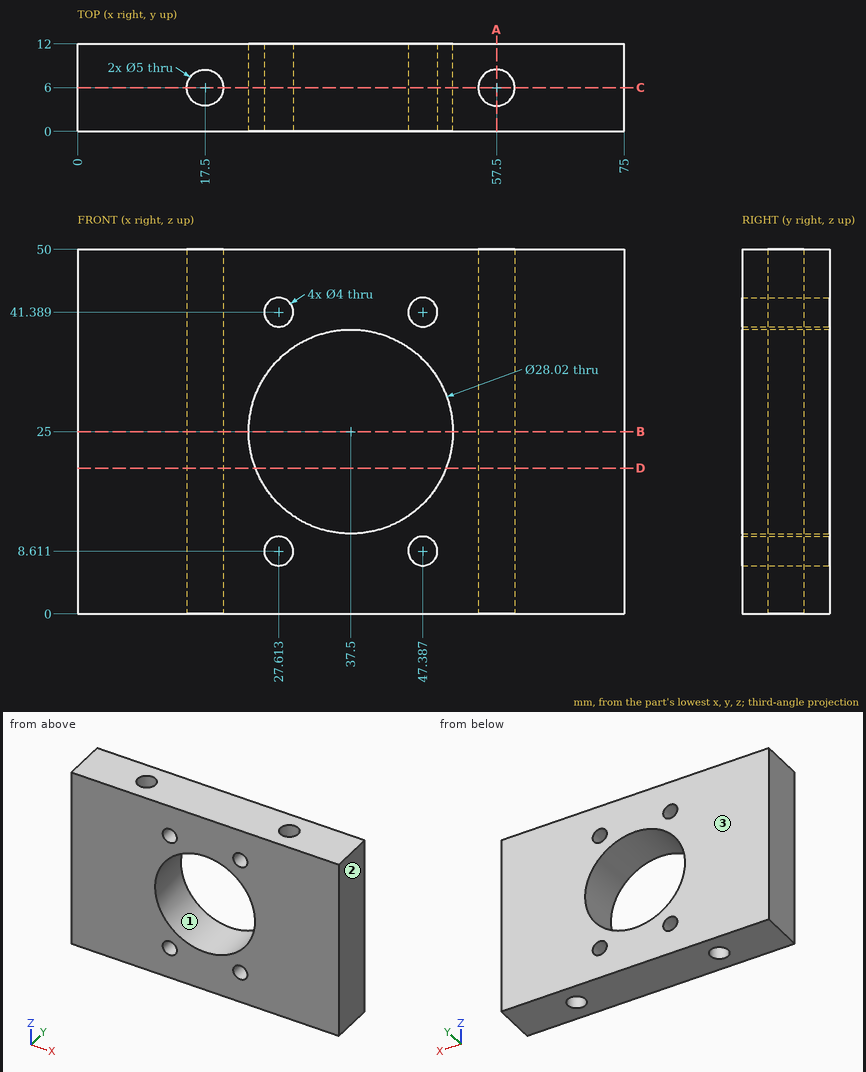
Geometry check sheet. Reference: drawing and pictorial views, mm from the part's lowest x, y, z. Round coordinates to 2 decimals unless told otherwise and drop trailing zeros. Loops run counter-clockwise (first coordinate to the right, second up) from the corner with the lowest first, then second, coordinate; pieces in that order, holes last. Notation, with made-up numbers: (34, 48.5) - (92, 48.5) arc R27 cw to (92, 82.5) - close; hole circle Ø9 at (-6.5, -33). An arc over 180 degrees is marked (long way). Answer in a Markdown table with one row per item. Add a question column.
Q1. Section check D-D on z = 20. Enter the section's corners in (x, y).
Q2. Release check for a two-part mould opening along X. For the marked faces 1, 2 and 3 record: pulls with the +X half, pulls with the -X half, needs draft (parallel to the pull), parting line crosses it, or undercut.
Q3. Material ranges on line 1 (X direction, y = 5.75, z = 4); line 2 (X direction, y = 11.25, z = 41.5); line 3 (X direction, y = 4.25, z = 27) (1 decimal), recorded low to high.
Q4. Section check B-B on z = 25. Enter the section's corners in (x, y).
Q5. Section check C-C on y = 6. Enter the section's corners in (x, z).
Q6. Section check A-A on x = 57.5. Enter the section's corners in (y, z), plus the area to 3 significant figures.
Found:
| question | item | result |
|---|---|---|
| 1 | outline | (0, 0) - (24.41, 0) - (24.41, 12) - (0, 12) - close; (50.59, 0) - (75, 0) - (75, 12) - (50.59, 12) - close; hole circle Ø5 at (17.5, 6); hole circle Ø5 at (57.5, 6) |
| 2 | face 1 | undercut |
| 2 | face 2 | pulls with the +X half |
| 2 | face 3 | needs draft |
| 3 | line 1 | x = 0 to 15.01, 19.99 to 55.01, 59.99 to 75 |
| 3 | line 2 | x = 0 to 25.62, 29.61 to 45.39, 49.38 to 75 |
| 3 | line 3 | x = 0 to 15.7, 19.3 to 23.6, 51.4 to 55.7, 59.3 to 75 |
| 4 | outline | (0, 0) - (23.49, 0) - (23.49, 12) - (0, 12) - close; (51.51, 0) - (75, 0) - (75, 12) - (51.51, 12) - close; hole circle Ø5 at (17.5, 6); hole circle Ø5 at (57.5, 6) |
| 5 | outline | (0, 0) - (15, 0) - (15, 50) - (0, 50) - close; (20, 0) - (55, 0) - (55, 50) - (20, 50) - close; (60, 0) - (75, 0) - (75, 50) - (60, 50) - close; hole circle Ø28.02 at (37.5, 25); hole circle Ø4 at (27.61, 8.61); hole circle Ø4 at (27.61, 41.39); hole circle Ø4 at (47.39, 8.61); hole circle Ø4 at (47.39, 41.39) |
| 6 | outline | (0, 0) - (3.5, 0) - (3.5, 50) - (0, 50) - close; (8.5, 0) - (12, 0) - (12, 50) - (8.5, 50) - close |
| 6 | area | 350 mm² |
